Geometry: final body of the model. Coordinates: model frame, mm. Give positions to 0.01 mm unless a question says otherwise; leave off trailing zeros. Order: outer loops, then holes, each group sorted by start corner. A loop starts at its lowest first (then second) coordinate and runs counter-clockwise, first axis right, second up. Notation, with made-up numbers: (33.5, 62) - (43.5, 62) arc R32 ccw to (43.5, 91) - close; hole circle Ø7 at (34, 54). An arc over 180 degrees is marked (long way). One line per item, written item: value.
```python
from build123d import *

# Parameters (mm, degrees)
SKETCH2_R               = 3.175
BOSS_EXTRUDE1_DEPTH     = 25.4
CHAMFER1_SIZE           = 0.254
SKETCH4_R               = 0.79375
CUT_EXTRUDE2_DEPTH      = 4.175
CUT_EXTRUDE2_DEPTH_BACK = 4.175


with BuildPart() as part:
    # Sketch2 → Boss-Extrude1 (new body)
    with BuildSketch(Plane(origin=(0, 0, 0), x_dir=(0, 0, -1), z_dir=(1, 0, 0))):
        Circle(SKETCH2_R)
    extrude(amount=BOSS_EXTRUDE1_DEPTH)

    # Chamfer1
    chamfer1_edges = [part.edges().sort_by_distance(p)[0] for p in [
        (0, 0, 3.175),
        (25.4, 0, 3.175),
    ]]
    chamfer(chamfer1_edges, length=CHAMFER1_SIZE)

    # Sketch4 → Cut-Extrude2 (cut, two sides)
    with BuildSketch(Plane(origin=(0, 0, 0), x_dir=(1, 0, 0), z_dir=(0, 1, 0))) as cut_extrude2_sk:
        with Locations((5.08, 0)):
            Circle(SKETCH4_R)
    extrude(amount=CUT_EXTRUDE2_DEPTH, mode=Mode.SUBTRACT)
    extrude(cut_extrude2_sk.sketch, amount=-CUT_EXTRUDE2_DEPTH_BACK, mode=Mode.SUBTRACT)


solid = part.part
```
1) Section A-A, the plane z = 0. Return loops of the section in (x, y) (3 decimals), then the cut area to 3 significant figures.
Answers below:
outline: (0, -2.921) - (0.254, -3.175) - (4.286, -3.175) - (4.286, 3.175) - (0.254, 3.175) - (0, 2.921) - close; (5.874, -3.175) - (25.146, -3.175) - (25.4, -2.921) - (25.4, 2.921) - (25.146, 3.175) - (5.874, 3.175) - close
area: 151 mm^2
2) Section B-B, the plane x = 3.25. Return loops of the section in (y, z) (3 decimals), then the cut area to 3 significant figures.
Answers below:
outline: circle Ø6.35 at (0, 0)
area: 31.7 mm^2
3) Mould query, pull axis Z, two halves, no side actions, for faces 1 (the face through (4.287, 0.044, -0.035)), 2 (the face through (25.4, 0, 0)), 3 (the face through (12.53, -3.1, 0.69)). Classes: released by +Z, released by -Z, zero draft, split by the parting line, or undercut.
Answers below:
face 1: undercut
face 2: zero draft
face 3: split by the parting line
4) Material intervals for line 1 along X through (y, z) = (0.5, 0); line 2 along Z through (x, y) = (5.08, 0.5); line 3 along Z through (x, y) = (15.5, -1.25), sorted ascending.
Answers below:
line 1: 0 to 4.29, 5.87 to 25.4
line 2: -3.14 to -0.79, 0.79 to 3.14
line 3: -2.92 to 2.92
